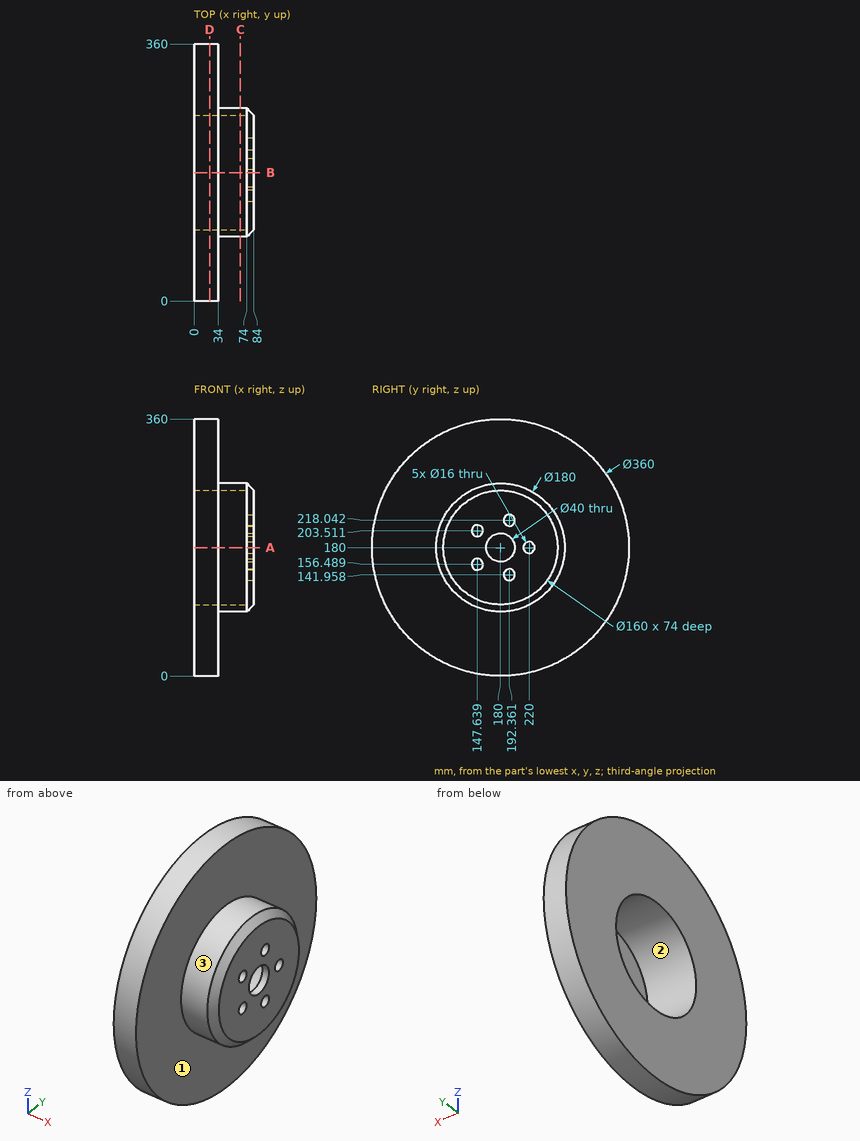
Geometry check sheet. Reference: drawing and pictorial views, mm from the part's lowest x, y, z. Give positions to 0.01 mm unless a question says otherwise; leave off trailing zeros. Write each loop counter-clockwise with the first axis right and the second up, starting at its lowest first coordinate (ties: lowest second). Pieces come first, ordered by that corner, then holes. Notation, with made-up numbers: M 84,-13 L 112,-13 A11 cw 112,-3 Z; hole C 43,33 d9. An arc over 180 degrees is marked long. Put each result on its own line as item: value. Start each with the question number.
1. Scan lines: line 1 along X through (y, z) = (184.5, 331); line 2 along Z through (x, y) = (45, 114); line 3 along Z through (x, y) = (77, 220). Record each from-to range of solid material in increasing order. Write a range as [from, to].
2. Section check B-B (y = 180). Record the cut outline in (x, z), and give its area (3 significant figures).
3. Draft check along Z on the marked faces 1, 2 and 3. Enter one of: +Z half, -Z half, draft (parallel to the pull), parting line (faces both ways), or undercut.
4. Section check C-C (x = 65). Record the cut outline in (y, z), and give its area (3 significant figures).
5. Section check A-A (z = 180). Record the cut outline in (x, y).
6. Go/stop test with flat-tipped pins: pin 1 Ø5 at (x, y) = (38, 248.5) entering from -Z; pin 2 Ø1 at (x, y) = (41.5, 196.5) entering from +Z; pin 3 Ø3 at (x, z) = (62.5, 192) entering from +Y (1 decimal). Record where each tip stops, or that it passes through.
7. Section check D-D (x = 22). Record the cut outline in (y, z), and give its area (3 significant figures).
Answer list:
1. line 1: [0, 34]
1. line 2: [118.81, 134.79], [225.21, 241.19]
1. line 3: [102.74, 172], [188, 257.26]
2. outline: M 0,0 L 34,0 L 34,90 L 74,90 L 84,100 L 84,160 L 74,160 L 74,100 L 0,100 Z; M 0,260 L 74,260 L 74,200 L 84,200 L 84,260 L 74,270 L 34,270 L 34,360 L 0,360 Z
2. area: 8,900 mm2
3. face 1: draft
3. face 2: undercut
3. face 3: parting line
4. outline: C 180,180 d180; hole C 180,180 d160
4. area: 5,340 mm2
5. outline: M 0,0 L 34,0 L 34,90 L 74,90 L 84,100 L 84,160 L 74,160 L 74,100 L 0,100 Z; M 0,260 L 74,260 L 74,228 L 84,228 L 84,260 L 74,270 L 34,270 L 34,360 L 0,360 Z; M 74,200 L 84,200 L 84,212 L 74,212 Z
6. pin 1: z = 118.81
6. pin 2: z = 268.57
6. pin 3: y = 269.4
7. outline: C 180,180 d360; hole C 180,180 d160
7. area: 81,700 mm2
